from build123d import *

# Parameters (mm, degrees)
SKETCH1_W           = 17.3
SKETCH1_H           = 20.6
SKETCH1_W_2         = 5.5
SKETCH1_H_2         = 3
BOSS_EXTRUDE1_DEPTH = 1.1
SKETCH2_W           = 11
SKETCH2_H           = 3
BOSS_EXTRUDE2_DEPTH = 3
SKETCH3_W           = 17.3
SKETCH3_H           = 20.6
SKETCH3_W_2         = 11
SKETCH3_H_2         = 3
BOSS_EXTRUDE3_DEPTH = 2


with BuildPart() as part:
    # Sketch1 → Boss-Extrude1 (new body)
    with BuildSketch(Plane.XY):
        with Locations((8.65, 10.3)):
            Rectangle(SKETCH1_W, SKETCH1_H)
        with Locations((20.05, 22.1)):
            Rectangle(SKETCH1_W_2, SKETCH1_H_2)
        with Locations((25.55, 22.1)):
            Rectangle(SKETCH1_W_2, SKETCH1_H_2)
        Polygon((28.3, 20.6), (22.8, 20.6), (17.3, 20.6), (17.3, 0), (22.8, 0), (28.3, 0), align=None)
        with Locations((36.95, 10.3)):
            Rectangle(SKETCH1_W, SKETCH1_H)
        with Locations((25.55, -1.5)):
            Rectangle(SKETCH1_W_2, SKETCH1_H_2)
        with Locations((20.05, -1.5)):
            Rectangle(SKETCH1_W_2, SKETCH1_H_2)
    extrude(amount=BOSS_EXTRUDE1_DEPTH)

    # Sketch2 → Boss-Extrude2 (add)
    with BuildSketch(Plane.XY.offset(1.1)):
        with Locations((22.8, 22.1)):
            Rectangle(SKETCH2_W, SKETCH2_H)
    extrude(amount=BOSS_EXTRUDE2_DEPTH)

    # Sketch3 → Boss-Extrude3 (add)
    with BuildSketch(Plane(origin=(0, 0, 0), x_dir=(-1, 0, 0), z_dir=(0, 0, -1))):
        with Locations((-36.95, 10.3)):
            Rectangle(SKETCH3_W, SKETCH3_H)
        with Locations((-22.8, 22.1)):
            Rectangle(SKETCH3_W_2, SKETCH3_H_2)
        with Locations((-22.8, 10.3)):
            Rectangle(SKETCH3_W_2, SKETCH3_H)
        with Locations((-8.65, 10.3)):
            Rectangle(SKETCH3_W, SKETCH3_H)
        with Locations((-22.8, -1.5)):
            Rectangle(SKETCH3_W_2, SKETCH3_H_2)
    extrude(amount=BOSS_EXTRUDE3_DEPTH)


solid = part.part
Check sheet for the modelled part. Datum: model origin and axes. Units: mm. A direction names the side the tool comes from. Round coordinates to 2 decimals unless told otherwise and drop trailing zeros. Loops run counter-clockwise (first coordinate to the right, second up) from the corner with the lowest first, then second, coordinate; pieces in that order, holes last. Notation, with made-up numbers: (79.25, 82) -> (89.25, 82) arc R36 cw to (89.25, 119) -> close; hole circle Ø7 at (11.5, 71.25). An arc over 180 degrees is marked (long way). Put each result on its own line as item: value. Start each with the question number.
1. Section check B-B (x = 25.5). Enter the section's corners in (y, z).
2. Section check C-C (y = 12). Enter the section's corners in (x, z).
3. Scan lines: probe 1 along Y at (x, z) = (23, 2.25); probe 2 along Z at (x, y) = (35, 11.75); probe 3 along Y at (x, z) = (43.5, -1.5). Record each from-to range of solid material in increasing order.
4. Section check D-D (x = 33.5). Enter the section's corners in (y, z).
5. Access from +Z, -Z, +X, -X, +Y, -Y to the whole of each face (thin tool, end or side, straight path). Record for faces 1 (the face through (17.3, 22, 1)), 2 (the face through (9, 0, 0)), 3 (the face through (28.3, -2, 0)), 4 (the face through (28.3, 22, 1)).
6. Gauge pin test, flat ends, axial feed: pin 1 (0.9 mm diameter, centred on x = 12.5, z = -0.5, fed in from +Y); pin 2 (1.5 mm diameter, centred on y = 22, z = 1, fed in from -X); pin 3 (3.5 mm diameter, centred on x = 41, z = 0, fed in from -Y). Record the tip position at first contact, or that the pin passes through.
7. Section check A-A (z = -1.25). Enter the section's corners in (x, y), plus the area to 3 significant figures.
Findings:
1. outline: (-3, -2) -> (23.6, -2) -> (23.6, 4.1) -> (20.6, 4.1) -> (20.6, 1.1) -> (-3, 1.1) -> close
2. outline: (0, -2) -> (45.6, -2) -> (45.6, 1.1) -> (0, 1.1) -> close
3. probe 1: y = 20.6 to 23.6
3. probe 2: z = -2 to 1.1
3. probe 3: y = 0 to 20.6
4. outline: (0, -2) -> (20.6, -2) -> (20.6, 1.1) -> (0, 1.1) -> close
5. face 1: +Z, -Z, -X, +Y
5. face 2: +Z, -Z, -X, -Y
5. face 3: +Z, -Z, +X, -Y
5. face 4: +Z, -Z, +X, +Y
6. pin 1: stops at y = 20.6
6. pin 2: stops at x = 17.3
6. pin 3: stops at y = 0
7. outline: (0, 0) -> (17.3, 0) -> (17.3, -3) -> (28.3, -3) -> (28.3, 0) -> (45.6, 0) -> (45.6, 20.6) -> (28.3, 20.6) -> (28.3, 23.6) -> (17.3, 23.6) -> (17.3, 20.6) -> (0, 20.6) -> close
7. area: 1,010 mm^2
